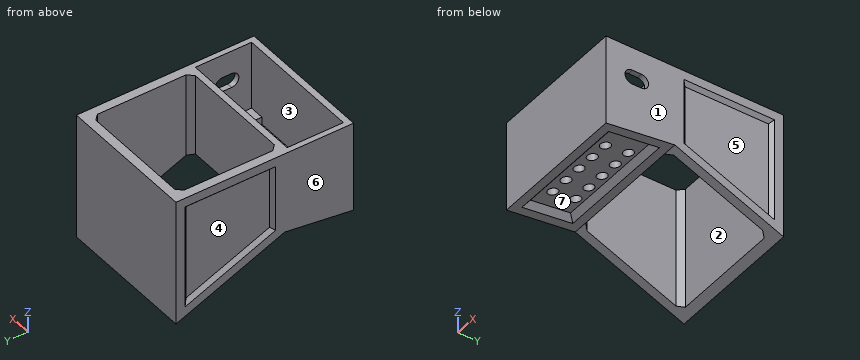
```python
from build123d import *

# Parameters (mm, degrees)
SKIZZE1_W                                   = 77
SKIZZE1_H                                   = 38
AUFSATZ_LINEAR_AUSTRAGEN1_DEPTH             = 25
SKIZZE5_R                                   = 2.75
SCHNITT_LINEAR_AUSTRAGEN1_DEPTH             = 66.903338307
SCHNITT_LINEAR_AUSTRAGEN2_DEPTH             = 50.681485485
SCHNITT_LINEAR_AUSTRAGEN2_DEPTH_BACK        = 50.681485485
SKIZZE8_W                                   = 67
SKIZZE8_H                                   = 28.327535794
SCHNITT_LINEAR_AUSTRAGEN8_DEPTH             = 3
SCHNITT_LINEAR_AUSTRAGEN8_DRAFT             = -45
SKIZZE9_W                                   = 71
SKIZZE9_H                                   = 31
SCHNITT_LINEAR_AUSTRAGEN9_DEPTH             = 50.681485485
SCHNITT_LINEAR_AUSTRAGEN9_DIRECTION_2_REACH = 51.681
AUFSATZ_LINEAR_START                        = -16.974828462
AUFSATZ_LINEAR_AUSTRAGEN2_OUTLINE_W         = 8
AUFSATZ_LINEAR_AUSTRAGEN2_OUTLINE_H         = 31
AUFSATZ_LINEAR_AUSTRAGEN2_DEPTH             = 4.078947369
AUFSATZ_LINEAR_AUSTRAGEN4_DEPTH             = 77
SKIZZE23_W                                  = 67
SKIZZE23_H                                  = 55
SCHNITT_LINEAR_AUSTRAGEN19_DEPTH            = 113.353237604
SCHNITT_LINEAR_AUSTRAGEN20_DEPTH            = 2
SCHNITT_LINEAR_AUSTRAGEN20_DRAFT            = -45
SPIEGELN9_COPY_1_DEPTH                      = 2
SPIEGELN9_COPY_1_DRAFT                      = -45
FASE2_SIZE                                  = 3
SCHNITT_LINEAR_AUSTRAGEN21_DEPTH            = 3


# Read off the part's stored shape, not the designer's step: Aufsatz-Linear austragen2
with BuildPart() as part:
    # Skizze1 → Aufsatz-Linear austragen1 (new, symmetric)
    with BuildSketch(Plane.XY):
        Rectangle(SKIZZE1_W, SKIZZE1_H)
    extrude(amount=AUFSATZ_LINEAR_AUSTRAGEN1_DEPTH, both=True)

    # Skizze5 → Schnitt-Linear austragen1 (cut, through all)
    with BuildSketch(Plane(origin=(0, 0, -25), x_dir=(-1, 0, 0), z_dir=(0, 0, -1))):
        with Locations((-20.32, 6.35)):
            Circle(SKIZZE5_R)
        with Locations((-20.32, -6.35)):
            Circle(SKIZZE5_R)
        with Locations((-10.16, 6.35)):
            Circle(SKIZZE5_R)
        with Locations((-10.16, -6.35)):
            Circle(SKIZZE5_R)
        with Locations((0, 6.35)):
            Circle(SKIZZE5_R)
        with Locations((0, -6.35)):
            Circle(SKIZZE5_R)
        with Locations((10.16, 6.35)):
            Circle(SKIZZE5_R)
        with Locations((10.16, -6.35)):
            Circle(SKIZZE5_R)
        with Locations((20.32, 6.35)):
            Circle(SKIZZE5_R)
        with Locations((20.32, -6.35)):
            Circle(SKIZZE5_R)
    extrude(amount=-SCHNITT_LINEAR_AUSTRAGEN1_DEPTH, mode=Mode.SUBTRACT)

    # Skizze6 → Schnitt-Linear austragen2 (cut, two sides: drawn at the far end of the back side and taken through both)
    with BuildSketch(Plane(origin=(0, 0, 0), x_dir=(0, 0, -1), z_dir=(1, 0, 0)).offset(-SCHNITT_LINEAR_AUSTRAGEN2_DEPTH_BACK)):
        Polygon((20, 19), (25, 19), (25, -19), align=None)
    extrude(amount=SCHNITT_LINEAR_AUSTRAGEN2_DEPTH + SCHNITT_LINEAR_AUSTRAGEN2_DEPTH_BACK, mode=Mode.SUBTRACT)


with BuildPart() as schnitt_linear_austragen8_tool:
    # Skizze8 → Schnitt-Linear austragen8 (with draft: the straight prism first)
    with BuildSketch(Plane(origin=(0, 2.910142954, -22.117086453), x_dir=(1, 0, 0), z_dir=(0, 0.1304545125713874, -0.9914542955425438))):
        with Locations((0, 2.935226533)):
            Rectangle(SKIZZE8_W, SKIZZE8_H)
    extrude(amount=-SCHNITT_LINEAR_AUSTRAGEN8_DEPTH)
    # Schnitt-Linear austragen8: the draft: its side faces are tilted about the plane it starts from
    schnitt_linear_austragen8_sides = [schnitt_linear_austragen8_tool.faces().sort_by_distance(p)[0] for p in [
        (-33.5, -0.195681769, -21.012818557),
        (0, 13.847046753, -19.16509112),
        (33.5, -0.195681769, -21.012818557),
        (0, -14.238410291, -22.860545994),
    ]]
    draft(schnitt_linear_austragen8_sides, Plane(origin=(0, 2.910142954, -22.117086453), x_dir=(1, 0, 0), z_dir=(0, 0.1304545125713874, -0.9914542955425438)), SCHNITT_LINEAR_AUSTRAGEN8_DRAFT)


with BuildPart() as part_1:
    add(part.part)

    # Schnitt-Linear austragen8: cut by schnitt_linear_austragen8_tool
    add(schnitt_linear_austragen8_tool.part, mode=Mode.SUBTRACT)

    # Skizze9 → Schnitt-Linear austragen9 (cut)
    with BuildSketch(Plane.XY):
        Rectangle(SKIZZE9_W, SKIZZE9_H)
    extrude(amount=SCHNITT_LINEAR_AUSTRAGEN9_DEPTH, mode=Mode.SUBTRACT)

    # Schnitt-Linear austragen9 direction 2: up to this plane
    schnitt_linear_austragen9_direction_2_end = Plane(origin=(0, 1.93173411, -14.681179237), z_dir=(0, 0.13045451257138746, -0.9914542955425438))
    # Skizze9 → Schnitt-Linear austragen9 direction 2 (cut, up to the surface)
    with BuildSketch(Plane.XY, mode=Mode.PRIVATE) as schnitt_linear_austragen9_direction_2_sk1:
        Rectangle(SKIZZE9_W, SKIZZE9_H)
    schnitt_linear_austragen9_direction_2_tool1 = split(extrude(schnitt_linear_austragen9_direction_2_sk1.sketch, amount=-SCHNITT_LINEAR_AUSTRAGEN9_DIRECTION_2_REACH, mode=Mode.PRIVATE), bisect_by=schnitt_linear_austragen9_direction_2_end, keep=Keep.BOTH, mode=Mode.PRIVATE)
    add(schnitt_linear_austragen9_direction_2_tool1.solids().sort_by_distance((0, 0, 0))[0], mode=Mode.SUBTRACT)

    # Aufsatz-Linear austragen2 outline → Aufsatz-Linear austragen2 (add)
    with BuildSketch(Plane.XY.offset(AUFSATZ_LINEAR_START)):
        with Locations((-31.5, 0)):
            Rectangle(AUFSATZ_LINEAR_AUSTRAGEN2_OUTLINE_W, AUFSATZ_LINEAR_AUSTRAGEN2_OUTLINE_H)
        with Locations((31.5, 0)):
            Rectangle(AUFSATZ_LINEAR_AUSTRAGEN2_OUTLINE_W, AUFSATZ_LINEAR_AUSTRAGEN2_OUTLINE_H)
    extrude(amount=AUFSATZ_LINEAR_AUSTRAGEN2_DEPTH)

    # Skizze22 → Aufsatz-Linear austragen4 (add)
    with BuildSketch(Plane(origin=(38.5, 0, 0), x_dir=(0, 0, -1), z_dir=(1, 0, 0))):
        Polygon((20, 19), (45, 79), (-25, 79), (-25, 19), align=None)
    extrude(amount=-AUFSATZ_LINEAR_AUSTRAGEN4_DEPTH)

    # Skizze23 → Schnitt-Linear austragen19 (cut, through all)
    with BuildSketch(Plane.XY.offset(25)):
        with Locations((0, 46.5)):
            Rectangle(SKIZZE23_W, SKIZZE23_H)
    extrude(amount=-SCHNITT_LINEAR_AUSTRAGEN19_DEPTH, mode=Mode.SUBTRACT)


with BuildPart() as schnitt_linear_austragen20_tool:
    # Skizze24 → Schnitt-Linear austragen20 (with draft: the straight prism first)
    with BuildSketch(Plane(origin=(38.5, 0, 0), x_dir=(0, 0, -1), z_dir=(1, 0, 0))):
        Polygon((16.666666667, 24), (37.5, 74), (-20, 74), (-20, 24), align=None)
    extrude(amount=-SCHNITT_LINEAR_AUSTRAGEN20_DEPTH)
    # Schnitt-Linear austragen20: the draft: its side faces are tilted about the plane it starts from
    schnitt_linear_austragen20_sides = [schnitt_linear_austragen20_tool.faces().sort_by_distance(p)[0] for p in [
        (37.5, 49, -27.083333333),
        (37.5, 74, -8.75),
        (37.5, 49, 20),
        (37.5, 24, 1.666666667),
    ]]
    draft(schnitt_linear_austragen20_sides, Plane(origin=(38.5, 0, 0), x_dir=(0, 0, -1), z_dir=(1, 0, 0)), SCHNITT_LINEAR_AUSTRAGEN20_DRAFT)


with BuildPart() as part_2:
    add(part_1.part)

    # Schnitt-Linear austragen20: cut by schnitt_linear_austragen20_tool
    add(schnitt_linear_austragen20_tool.part, mode=Mode.SUBTRACT)


with BuildPart() as spiegeln9_copy_1_tool:
    # Spiegeln9 copy 1 sketch → Spiegeln9 copy 1 (with draft: the straight prism first)
    with BuildSketch(Plane(origin=(-38.5, 0, 0), x_dir=(0, 0, -1), z_dir=(-1, 0, 0))):
        Polygon((16.666666667, -24), (37.5, -74), (-20, -74), (-20, -24), align=None)
    extrude(amount=-SPIEGELN9_COPY_1_DEPTH)
    # Spiegeln9 copy 1: the draft: its side faces are tilted about the plane it starts from
    spiegeln9_copy_1_sides = [spiegeln9_copy_1_tool.faces().sort_by_distance(p)[0] for p in [
        (-37.5, 49, -27.083333333),
        (-37.5, 74, -8.75),
        (-37.5, 49, 20),
        (-37.5, 24, 1.666666667),
    ]]
    draft(spiegeln9_copy_1_sides, Plane(origin=(-38.5, 0, 0), x_dir=(0, 0, -1), z_dir=(-1, 0, 0)), SPIEGELN9_COPY_1_DRAFT)


with BuildPart() as part_3:
    add(part_2.part)

    # Spiegeln9 copy 1: cut by spiegeln9_copy_1_tool
    add(spiegeln9_copy_1_tool.part, mode=Mode.SUBTRACT)

    # Fase2
    fase2_edges = [part_3.edges().sort_by_distance(p)[0] for p in [
        (33.5, 74, -8.958333333),
        (33.5, 19, 2.5),
        (-33.5, 19, 2.5),
        (-33.5, 74, -8.958333333),
    ]]
    chamfer(fase2_edges, length=FASE2_SIZE)

    # Skizze25 → Schnitt-Linear austragen21 (cut)
    with BuildSketch(Plane.ZY.offset(-35.5)):
        with BuildLine():
            Line((4.104118907, -4.5), (4.104118907, 0.5))
            ThreePointArc((4.104118907, 0.5), (8.104118907, 4.5), (12.104118907, 0.5))
            Line((12.104118907, 0.5), (12.104118907, -4.5))
            ThreePointArc((12.104118907, -4.5), (8.104118907, -8.5), (4.104118907, -4.5))
        make_face()
    extrude(amount=-SCHNITT_LINEAR_AUSTRAGEN21_DEPTH, mode=Mode.SUBTRACT)


solid = part_3.part
```
Input: part model. Units: mm. Frame: model coordinates. Face numbers are marked on the shaded views. A direction names the side the tool comes from. Round coordinates to 2 decimals unless told otherwise and drop trailing zeros. Loops run counter-clockwise (first coordinate to the right, second up) from the corner with the lowest first, then second, coordinate; pieces in that order, holes last. Notation, with made-up numbers: (57, 68) - (114, 68) arc R15 cw to (114, 78) - close; hole circle Ø1 at (51.5, 5). An arc over 180 degrees is marked (long way). One line per item, written item: value. Start each with the question number.
(1) Section B-B, the plane y = 30. Return loops of the section in (x, z).
(2) Contact query for flat-ended pins moving along their axis: P1, Ø6.5, axis at x = -10.16, y = 6.35, coming from the +Z side; P2, Ø7, axis at x = 0, y = -6.35, coming from the +Z side; P3, Ø9, axis at x = 0, y = 6.35, coming from the +Z side; P4, Ø25, axis at y = -0.5, z = 4.5, coming from the +X side. Output: stop coordinate, or through.
(3) Section C-C, the plane x = 20.32. Return loops of the section in (y, z).
(4) Ray query, line 1 (X direction, y = -6.35, z = -19.4); line 2 (Y direction, x = 20.32, z = -17.8); line 3 (Y direction, x = -3.5, z = -8.5). Return the intervals inside material, ascending. Write a range as [from, to].
(5) Draft query along Z for the marked faces 5, 6 and 7. Return one class per face: +Z half, -Z half, draft (parallel to the pull), parting line (faces both ways), or undercut.
(6) Section D-D, the plane z = 10. Return loops of the section in (x, y), plus the area to 3 significant figures.
(7) Access query for the marked faces 1, 2, 3 and 4. Directions: +Z, -Z, +X, -X, +Y, -Y. A direction counts if a zero-diameter tool reaches every point of the face in a straight line with its end or side. Return the directions, or none.
(8) Section A-A, the plane z = 2. Return loops of the section in (x, y).
Results below:
1. outline: (-38.5, -24.58) - (-33.5, -24.58) - (-33.5, 25) - (-38.5, 25) - (-38.5, 20) - (-36.5, 18) - (-36.5, -17) - (-38.5, -19.17) - close; (33.5, -24.58) - (38.5, -24.58) - (38.5, -19.17) - (36.5, -17) - (36.5, 18) - (38.5, 20) - (38.5, 25) - (33.5, 25) - close
2. P1: z = -13.67
2. P2: z = -15.31
2. P3: z = -13.51
2. P4: x = 38.5
3. outline: (-19, -25) - (-14.04, -24.35) - (-11.46, -20.98) - (-9.1, -20.67) - (-9.1, -16.13) - (-15.5, -16.97) - (-15.5, 25) - (-19, 25) - close; (-3.6, -19.95) - (3.6, -19) - (3.6, -14.46) - (-3.6, -15.41) - close; (9.1, -18.28) - (10.68, -18.07) - (14.04, -20.65) - (19, -20) - (19, 25) - (15.5, 25) - (15.5, -12.9) - (9.1, -13.74) - close; (74, -42.92) - (79, -45) - (79, 25) - (74, 25) - close
4. line 1: [-38.5, -23.07], [-17.57, -12.91], [-7.41, -2.75], [2.75, 7.41], [12.91, 17.57], [23.07, 38.5]
4. line 2: [-19, -9.1], [-3.6, 3.6], [9.1, 19], [74, 79]
4. line 3: [-19, -15.5], [15.5, 19], [74, 79]
5. face 5: undercut
5. face 6: draft
5. face 7: -Z half
6. outline: (-38.5, -19) - (38.5, -19) - (38.5, -8.02) - (35.5, -8.02) - (35.5, -15.5) - (-35.5, -15.5) - (-35.5, 15.5) - (35.5, 15.5) - (35.5, 4.02) - (38.5, 4.02) - (38.5, 24) - (36.5, 26) - (36.5, 72) - (38.5, 74) - (38.5, 79) - (-38.5, 79) - (-38.5, 74) - (-36.5, 72) - (-36.5, 26) - (-38.5, 24) - close; hole (-33.5, 22) - (-30.5, 19) - (30.5, 19) - (33.5, 22) - (33.5, 71) - (30.5, 74) - (-30.5, 74) - (-33.5, 71) - close
6. area: 1,450 mm^2
7. face 1: +Z, -Z, +X, +Y, -Y
7. face 2: +Z, -Z
7. face 3: +Z
7. face 4: -X
8. outline: (-38.5, -19) - (38.5, -19) - (38.5, 24) - (36.5, 26) - (36.5, 72) - (38.5, 74) - (38.5, 79) - (-38.5, 79) - (-38.5, 74) - (-36.5, 72) - (-36.5, 26) - (-38.5, 24) - close; hole (-35.5, -15.5) - (35.5, -15.5) - (35.5, 15.5) - (-35.5, 15.5) - close; hole (-33.5, 22) - (-30.5, 19) - (30.5, 19) - (33.5, 22) - (33.5, 71) - (30.5, 74) - (-30.5, 74) - (-33.5, 71) - close
